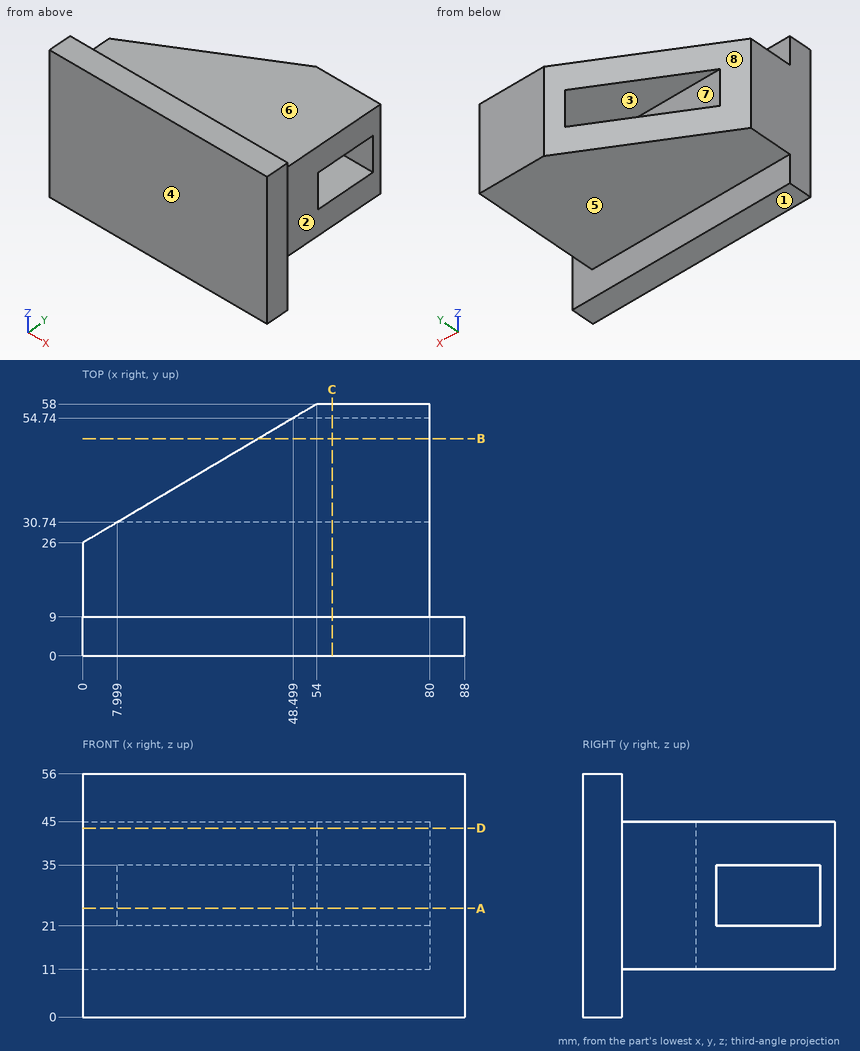
Input: dimensioned drawing with shaded views. Units: mm. Origin: part minimum x, y, z. A direction names the side the tool comes from. Coordinates: 2 decimals unless noted, no trailing zeros. Loops run counter-clockwise (first coordinate to the right, second up) from the corner with the lowest first, then second, coordinate; pieces in that order, holes last. Notation, with made-up numbers: (-36.75, 75.5) -> (18.25, 75.5) arc R24 cw to (18.25, 90.5) -> close; hole circle Ø7 at (8.25, 89.5). An arc over 180 degrees is marked (long way). Use a Markdown table: item, result. Add a question column.
(1) Section query A-A, the plane z = 25. Return loops of the section in (x, y), plus the area to 3 significant figures.
(2) Pin query (flat end, axial travel): pin 1 Ø2 at (y, z) = (32, 39) entering from +X; pin 2 Ø4 at (x, z) = (66, 30) entering from -Y; pin 3 Ø12 at (x, y) = (54.5, 47.5) entering from +Z; pin 4 Ø14.5 at (x, y) = (43, 35.5) entering from -Z. Return the tip coordinate at first contact, or that it passes through.
(3) Section query D-D, the plane z = 43.5. Return loops of the section in (x, y).
(4) Line query: line 1 along Z through (x, y) = (40, 31.5); line 2 along Y through (x, z) = (57, 7); line 3 along Z through (x, y) = (28, 25). Output: solid intervals per line, ascending.
(5) Section query C-C, the plane x = 57.5. Return loops of the section in (y, z).
(6) Section query B-B, the plane y = 50. Return loops of the section in (x, z).
(7) Access query for the marked faces 1, 2, 3, 4 and 5. Directions: +Z, -Z, +X, -X, +Y, -Y. A direction counts if a zero-diameter tool reaches every point of the face in a straight line with its end or side. Return the directions, or none.
(8) Mould query, pull axis Y, two halves, no side actions, for the marked faces 6, 7 and 8. Classes: pulls with the +Y half, pulls with the -Y half, needs draft (parallel to the pull), parting line crosses it, or undercut.
Answer:
| question | item | result |
|---|---|---|
| 1 | outline | (0, 0) -> (88, 0) -> (88, 9) -> (80, 9) -> (80, 30.74) -> (8, 30.74) -> (0, 26) -> close; (48.5, 54.74) -> (80, 54.74) -> (80, 58) -> (54, 58) -> close |
| 1 | area | 2,610 mm^2 |
| 2 | pin 1 | stops at x = 80 |
| 2 | pin 2 | stops at y = 0 |
| 2 | pin 3 | stops at z = 45 |
| 2 | pin 4 | stops at z = 11 |
| 3 | outline | (0, 0) -> (88, 0) -> (88, 9) -> (80, 9) -> (80, 58) -> (54, 58) -> (0, 26) -> close |
| 4 | line 1 | z = 11 to 21, 35 to 45 |
| 4 | line 2 | y = 0 to 9 |
| 4 | line 3 | z = 11 to 45 |
| 5 | outline | (0, 0) -> (9, 0) -> (9, 11) -> (58, 11) -> (58, 45) -> (9, 45) -> (9, 56) -> (0, 56) -> close; hole (30.74, 21) -> (54.74, 21) -> (54.74, 35) -> (30.74, 35) -> close |
| 6 | outline | (40.5, 11) -> (80, 11) -> (80, 21) -> (40.5, 21) -> close; (40.5, 35) -> (80, 35) -> (80, 45) -> (40.5, 45) -> close |
| 7 | face 1 | -Z, +X, -X, +Y, -Y |
| 7 | face 2 | +Z, -Z, +X, +Y |
| 7 | face 3 | +X, -X |
| 7 | face 4 | +Z, -Z, +X, -X, -Y |
| 7 | face 5 | -Z, +X, -X, +Y |
| 8 | face 6 | needs draft |
| 8 | face 7 | undercut |
| 8 | face 8 | pulls with the +Y half |
